Work out the finished part from the listing and answer in its coordinate system (mm). A direction names the side the tool comes from. Give positions to 0.01 mm unless a question says otherwise; leave off trailing zeros. Loops run counter-clockwise (first coordinate to the right, second up) from the corner with the lowest first, then second, coordinate; pieces in that order, holes last. Notation, with made-up numbers: (-20, 0.5) - (37, 0.5) arc R19 ccw to (37, 18.5) - close; hole circle Ø11 at (-23.75, -38.5). An arc over 180 degrees is marked (long way). Use CSV: the item, a comma, the result in double quotes.
from build123d import *

# Parameters (mm, degrees)
SKETCH1_W           = 70
SKETCH1_H           = 70
SKETCH1_W_2         = 64
SKETCH1_H_2         = 64
BOSS_EXTRUDE1_DEPTH = 860
FILLET1_R           = 5


with BuildPart() as part:
    # Sketch1 → Boss-Extrude1 (new body)
    with BuildSketch(Plane(origin=(0, 0, 0), x_dir=(1, 0, 0), z_dir=(0, 1, 0))):
        with Locations((35, 35)):
            Rectangle(SKETCH1_W, SKETCH1_H)
        with Locations((35, 35)):
            Rectangle(SKETCH1_W_2, SKETCH1_H_2, mode=Mode.SUBTRACT)
    extrude(amount=BOSS_EXTRUDE1_DEPTH)

    # Fillet1
    fillet1_edges = [part.edges().sort_by_distance(p)[0] for p in [
        (3, 430, -67),
        (3, 430, -3),
        (67, 430, -3),
        (67, 430, -67),
        (0, 430, 0),
        (0, 430, -70),
        (70, 430, -70),
        (70, 430, 0),
    ]]
    fillet(fillet1_edges, radius=FILLET1_R)


solid = part.part
Item 1: The mould has two halves that part along X. Classify faces 1 (the flat face through (0, 424, -35)), 2 (the flat face through (32, 0, -1)), 3 (the flat face through (70, 424, -35)), 4 (the flat face through (67, 424, -35)): pulls with the +X half, pulls with the -X half, needs draft (parallel to the pull), parting line crosses it, or undercut.
Determined:
face 1,"pulls with the -X half"
face 2,"needs draft"
face 3,"pulls with the +X half"
face 4,"undercut"
Item 2: For faces 5 (the flat face through (32, 860, -1)), 6 (the flat face through (3, 424, -35)), determine the directions among +Z, -Z, +X, -X, +Y, -Y from which every point of the face is accessible in a straight line to the end or side of a thin tool.
Determined:
face 5,"+Z, -Z, +X, -X, +Y"
face 6,"+Y, -Y"
Item 3: A cutting plane is placed at C-C on y = 614.5. Determine the outline of the cut face in (x, z).
Determined:
outline,"(0, -65) arc R5 ccw to (5, -70) - (65, -70) arc R5 ccw to (70, -65) - (70, -5) arc R5 ccw to (65, 0) - (5, 0) arc R5 ccw to (0, -5) - close; hole (3, -62) arc R5 ccw to (8, -67) - (62, -67) arc R5 ccw to (67, -62) - (67, -8) arc R5 ccw to (62, -3) - (8, -3) arc R5 ccw to (3, -8) - close"
Item 4: A cutting plane is placed at B-B on x = 31.5. Determine the outline of the cut face in (y, z).
Determined:
outline,"(0, -70) - (860, -70) - (860, -67) - (0, -67) - close; (0, -3) - (860, -3) - (860, 0) - (0, 0) - close"
Item 5: Find the intervals of material crossed by line 1 (Z direction, x = 45, y = 434); line 2 (X direction, y = 62.5, z = -21); line 3 (Z direction, x = 5, y = 460.5), in increasing order.
Determined:
line 1,"z = -70 to -67, -3 to 0"
line 2,"x = 0 to 3, 67 to 70"
line 3,"z = -70 to -66, -4 to 0"
Item 6: A cutting plane is placed at A-A on z = -44.5. Determine the outline of the cut face in (x, y), and give its area (3 significant figures).
Determined:
outline,"(0, 0) - (3, 0) - (3, 860) - (0, 860) - close; (67, 0) - (70, 0) - (70, 860) - (67, 860) - close"
area,"5,160 mm²"
